Autodesk Inventor part; units mm, degrees
ref_plane "YZ Plane" through (0, 0, 0) normal (1, 0, 0) x (0, 1, 0)
ref_plane "XZ Plane" through (0, 0, 0) normal (0, 1, 0) x (-1, 0, 0)
ref_plane "XY Plane" through (0, 0, 0) normal (0, 0, 1) x (1, 0, 0)
sketch "Sketch1" plane through (0, 0, 0) normal (0, 1, 0) x (-1, 0, 0)
  circle A0 centre (0, 0) radius 8.575
extrude "Extrusion1" add sketch "Sketch1" along normal blind 20
sketch "Sketch2" plane through (0, 20, 0) normal (0, 1, 0) x (1, 0, 0)
  circle A0 centre (0, 0) radius 8.575
  circle A1 centre (0, 0) radius 10.575
extrude "Extrusion2" add sketch "Sketch2" against normal blind 4
sketch "Sketch3" plane through (0, 20, 0) normal (0, 1, 0) x (1, 0, 0)
  circle A0 centre (0, 0) radius 10.575
  circle A1 centre (0, 0) radius 6.94
extrude "Extrusion3" cut sketch "Sketch3" against normal through all contours A1
fillet "Fillet1" radius 1 4 edges at (-10.575, 20, 0) (-6.94, 20, 0) (-10.575, 16, 0) (8.575, 0, 0)
properties part number "flaskPort"
Here's how the part is built. I have some questions about the finished solid (model axes, mm). A direction names the side the tool comes from. Give positions to 0.01 mm unless a question says otherwise; leave off trailing zeros. Order: outer loops, then holes, each group sorted by start corner. A loop starts at its lowest first (then second) coordinate and runs counter-clockwise, first axis right, second up. Notation, with made-up numbers: M 52,-13 L 75,-13 A20 cw 75,19 Z; hole C -2,64.5 d5. An arc over 180 degrees is marked long. Use a Markdown table: item, result. Add a question column.
1. Suppose I cut it at C-C (y = 7.25). List the corners of the cut face in (x, z) for me (3 decimals).
2. On a 3-axis mill with a long thin cutter (end or side, diameter ignored), from which of +Z, -Z, +X, -X, +Y, -Y can I reach the whole of each face in a straight line? I mean faces 4 (the flat face through (-9, 16, -1)), 5 (the cylindrical face through (-2.292, 18.014, 10.324)). Say none if no direction works.
3. If we mould it in two halves opening along X, with no side actions, what happens to faces 1 (the cylindrical face through (6.62, 9.63, -2.08)), 2 (the flat face through (-2, 0, -7)), 3 (the cylindrical face through (-8.179, 8.395, -2.576))? For each: +X half, -X half, draft (parallel to the pull), parting line (faces both ways), or undercut.
4. Suppose I cut it at B-B (x = 0). List the corners of the cut face in (y, z) for me (3 decimals).
5. I need wall thicknesses on probe 1 along Z at (x, y) = (0, 11) (3 decimals); probe 2 along X at (y, z) = (17.25, -0.25). Which ranges of each line are inside material? Lowest first, please. Write a range as from..to.
6. For pin 1 Ø12 at (y, z) = (16, 7) entering from +X; pin 2 Ø8 at (x, y) = (3, 10) entering from +Z (3 decimals); pin 3 Ø1 at (x, z) = (7.5, -8.5) entering from +Y; pin 4 Ø4 at (y, z) = (3, 1) entering from +X (3 decimals), each with a flat end and sliding along its axis, tell me the tip position at first contact or that it passes through.
7. Suppose I cut it at A-A (z = 0). List the corners of the cut face in (x, y) for me (3 decimals), and give its area (3 significant figures).
Results list:
| question | item | result |
|---|---|---|
| 1 | outline | C 0,0 d17.15; hole C 0,0 d13.88 |
| 2 | face 4 | -Y |
| 2 | face 5 | +Y, -Y |
| 3 | face 1 | undercut |
| 3 | face 2 | draft |
| 3 | face 3 | parting line |
| 4 | outline | M 0,-7.575 A1 ccw 1,-8.575 L 16,-8.575 L 16,-9.575 A1 ccw 17,-10.575 L 19,-10.575 A1 ccw 20,-9.575 L 20,-7.94 A1 ccw 19,-6.94 L 0,-6.94 Z; M 0,6.94 L 19,6.94 A1 ccw 20,7.94 L 20,9.575 A1 ccw 19,10.575 L 17,10.575 A1 ccw 16,9.575 L 16,8.575 L 1,8.575 A1 ccw 0,7.575 Z |
| 5 | probe 1 | z = -8.575..-6.94, 6.94..8.575 |
| 5 | probe 2 | x = -10.57..-6.94, 6.94..10.57 |
| 6 | pin 1 | stops at x = 10.52 |
| 6 | pin 2 | stops at z = 8.575 |
| 6 | pin 3 | passes through |
| 6 | pin 4 | stops at x = 8.575 |
| 7 | outline | M -10.575,17 A1 ccw -9.575,16 L -8.575,16 L -8.575,1 A1 ccw -7.575,0 L -6.94,0 L -6.94,19 A1 ccw -7.94,20 L -9.575,20 A1 ccw -10.575,19 Z; M 6.94,0 L 7.575,0 A1 ccw 8.575,1 L 8.575,16 L 9.575,16 A1 ccw 10.575,17 L 10.575,19 A1 ccw 9.575,20 L 7.94,20 A1 ccw 6.94,19 Z |
| 7 | area | 79.7 mm² |
